Drawing for the job (mm, zero at the part's lowest x, y, z). Coordinates: 2 decimals unless noted, no trailing zeros. Write each loop counter-clockwise with the first axis right and the second up, starting at its lowest first coordinate (ties: lowest second). Pieces come first, ordered by that corner, then holes. Notation, with made-up numbers: (75.25, -31) - (83.25, -31) arc R36 cw to (83.25, 5) - close; hole circle Ø2 at (32.5, 72.25). An arc over 180 degrees is marked (long way). Write each question's results on one line, items separated by ' | '.
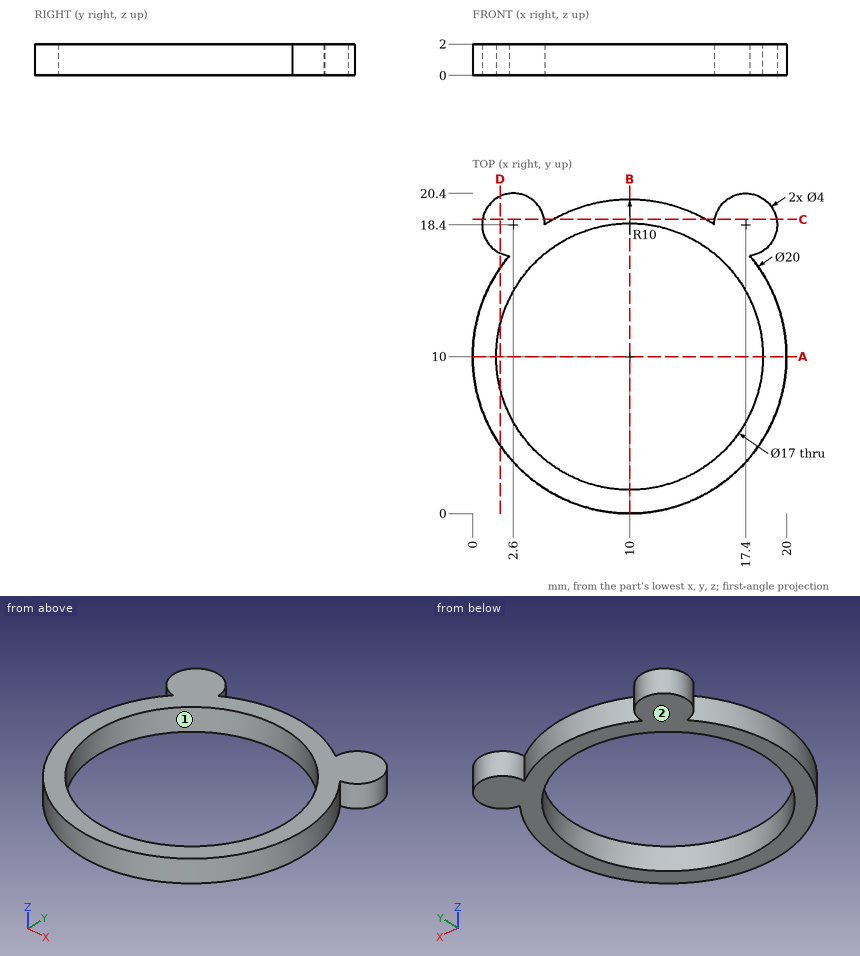
(1) Two-plate mould, pull along X, no slides. Class the marked faces 1 and 2: released by +X, released by -X, zero draft, split by the parting line, or undercut.
Return value:
face 1: undercut | face 2: zero draft
(2) Wall check: line 1 (Y direction, x = 10, z = 0.55); line 2 (Y direction, x = 6, z = 0.6). Give the ranges that are in metal, low to high. Write a range as from..to.
Return value:
line 1: y = 0..1.5, 18.5..20 | line 2: y = 0.83..2.5, 17.5..19.17
(3) Saw through at D-D on x = 1.75. Write the cut outline in (y, z), then the cut area to 3 significant figures.
Return value:
outline: (4.35, 0) - (7.95, 0) - (7.95, 2) - (4.35, 2) - close; (12.05, 0) - (15.65, 0) - (15.65, 2) - (12.05, 2) - close; (16.59, 0) - (20.21, 0) - (20.21, 2) - (16.59, 2) - close | area: 21.7 mm^2
(4) Saw through at A-A on y = 10. Write the cut outline in (x, z).
Return value:
outline: (0, 0) - (1.5, 0) - (1.5, 2) - (0, 2) - close; (18.5, 0) - (20, 0) - (20, 2) - (18.5, 2) - close
(5) Saw through at C-C on y = 18.75. Write the cut outline in (x, z), then the cut area to 3 significant figures.
Return value:
outline: (0.63, 0) - (4.57, 0) - (4.57, 2) - (0.63, 2) - close; (5.16, 0) - (14.84, 0) - (14.84, 2) - (5.16, 2) - close; (15.43, 0) - (19.37, 0) - (19.37, 2) - (15.43, 2) - close | area: 35.1 mm^2
